Here's how the part is built. I have some questions about the finished solid (model axes, mm). A direction names the side the tool comes from. Give positions to 0.01 mm unless a question says otherwise; leave off trailing zeros. Loops run counter-clockwise (first coordinate to the right, second up) from the corner with the lowest first, then second, coordinate; pieces in that order, holes last. Notation, with made-up numbers: M -23.5,-2 L -9.5,-2 A25 cw -9.5,11 Z; hole C -22,-27.75 d8. An arc over 180 degrees is marked long. Answer as CSV lines item,"result". Start each with the question number.
Item 1: I want a section at B-B on y = -30.5. List the corners of the cut face in (x, z) for me, plus the area to 3 significant figures.
Item 2: I want a section at A-A on z = 17. List the corners of the cut face in (x, y) for me, plus the area to 3 significant figures.
Item 3: I want a section at D-D on x = -5. List the corners of the cut face in (y, z) for me.
Item 4: If I drill on line 1 along X through (y, z) = (-43, 4.5); line 2 along X through (y, z) = (-29.5, 17); line 3 along Z through (x, y) = (86.5, -67), over which ranges is the centre line in solid material (lowest first)? Write a range as from..to.
Item 5: If we mould it in two halves opening along X, with no side actions, what happens to faces 5 (the flat face through (114.1, -63.3, 6.4)), 6 (the flat face through (52, -38, 50.8)), 7 (the flat face through (12.7, -38, 9)), 8 (the flat face through (50, -38, 19.05))? For each: released by +X, released by -X, zero draft, split by the parting line, or undercut.
Item 6: Will these pins go through, and if not, where does the flat tip stop? P1, Ø6, axis at y = -29, z = 40, coming from the -X side; P2, Ø3, axis at y = -44, z = 21.5, coming from the +X side; P3, Ø12.5, axis at x = -8.5, y = -36, coming from the +Z side; P4, Ø6, axis at x = -9.5, y = -45.5, coming from the -Z side.
Item 7: I want a section at C-C on z = 7.5. List the corners of the cut face in (x, y) for me.
Item 8: For faces 1 (the flat face through (0, -38, 32)), 2 (the flat face through (114, -13, 6)), 3 (the flat face through (111, -10, 12.7)), 4 (the flat face through (88.9, -38, 10)), which set-ups out of +Z, -Z, +X, -X, +Y, -Y let a thin tool reach every point of the face, with its end or its side?
from build123d import *

# Parameters (mm, degrees)
F1_DEPTH = 76.2
F0_W     = 25.4
F0_H     = 12.7
F2_DEPTH = 76.2
F4_DEPTH = 25.4


with BuildPart() as f1:
    # F0 (on Front) → F1 (new body)
    with BuildSketch(Plane.XZ):
        Polygon((-25.4, 0), (0, 0), (12.7, 0), (12.7, 19.05), (88.9, 19.05), (88.9, 0), (101.6, 0), (101.6, 12.7), (101.6, 50.8), (0, 50.8), (0, 12.7), (-25.4, 12.7), align=None)
    extrude(amount=F1_DEPTH)

    # F0 (on Front) → F2 (join)
    with BuildSketch(Plane.XZ):
        with Locations((114.3, 6.35)):
            Rectangle(F0_W, F0_H)
    extrude(amount=F2_DEPTH)

    # F3 (on face) → F4 (cut)
    with BuildSketch(Plane.XY.offset(12.7)):
        Polygon((101.6, -25.4), (101.6, -50.8), (127, -76.2), (127, 0), align=None)
    extrude(amount=-F4_DEPTH, mode=Mode.SUBTRACT)


solid = f1.part
Result:
1,outline,"M -25.4,0 L 12.7,0 L 12.7,19.05 L 88.9,19.05 L 88.9,0 L 101.6,0 L 101.6,50.8 L 0,50.8 L 0,12.7 L -25.4,12.7 Z"
1,area,"4,030 mm^2"
2,outline,"M 0,-76.2 L 12.7,-76.2 L 12.7,0 L 0,0 Z; M 88.9,-76.2 L 101.6,-76.2 L 101.6,0 L 88.9,0 Z"
2,area,"1,940 mm^2"
3,outline,"M -76.2,0 L 0,0 L 0,12.7 L -76.2,12.7 Z"
4,line 1,"-25.4..12.7, 88.9..101.6"
4,line 2,"0..12.7, 88.9..101.6"
4,line 3,"19.05..50.8"
5,face 5,"released by +X"
5,face 6,"zero draft"
5,face 7,"undercut"
5,face 8,"undercut"
6,P1,"x = 0"
6,P2,"x = 101.6"
6,P3,"z = 12.7"
6,P4,"z = 0"
7,outline,"M -25.4,-76.2 L 12.7,-76.2 L 12.7,0 L -25.4,0 Z; M 88.9,-76.2 L 127,-76.2 L 101.6,-50.8 L 101.6,-25.4 L 127,0 L 88.9,0 Z"
8,face 1,"+Z, -X, +Y, -Y"
8,face 2,"+Z, -Z, +X"
8,face 3,"+Z, +X, +Y, -Y"
8,face 4,"-Z, +Y, -Y"
